Design review of the part built by this model. Coordinates are the model's own, in mm. A direction names the side the tool comes from. Round coordinates to 2 decimals unless told otherwise and drop trailing zeros. Order: outer loops, then holes, each group sorted by start corner. A loop starts at its lowest first (then second) coordinate and runs counter-clockwise, first axis right, second up. Notation, with made-up numbers: (57, 7) - (83, 7) arc R15 cw to (83, 28) - close; hole circle Ø3 at (60.25, 73). An arc over 180 degrees is marked (long way). Write item = value, one per line.
from build123d import *

# Parameters (mm, degrees)
F0_R     = 12.7
F0_R_2   = 11.176
F1_DEPTH = 7


with BuildPart() as f1:
    # F0 (on Top) → F1 (new body)
    with BuildSketch(Plane.XY):
        with BuildLine():
            Line((-34.0347428799, 10.0407234107), (-39.4287826318, 25.8310334972))
            ThreePointArc((-39.4287826318, 25.8310334972), (-49.9900963881, -1.1227458082), (-41.9203568823, -28.9243081997))
            Line((-41.9203568823, -28.9243081997), (-34.420360506, -14.0186176143))
            Line((-34.420360506, -14.0186176143), (-29.2602696984, -22.6658631364))
            Line((-29.2602696984, -22.6658631364), (-26.4620529027, -14.6181120741))
            ThreePointArc((-26.4620529027, -14.6181120741), (-14.1637665374, -14.9822916534), (-4.52611316, -22.6305667311))
            ThreePointArc((-4.52611316, -22.6305667311), (-1.6908403761, -25.8780046014), (-0.1272074495, -29.8954262311))
            ThreePointArc((-0.1272074495, -29.8954262311), (1.2367097468, -25.698504913), (3.97388684, -22.2369618714))
            ThreePointArc((3.97388684, -22.2369618714), (12.644433264, -15.5734140078), (23.5379470973, -14.6181120741))
            Line((23.5379470973, -14.6181120741), (25.7397303016, -22.8490576527))
            Line((25.7397303016, -22.8490576527), (30.579639494, -14.0186176143))
            Line((30.579639494, -14.0186176143), (38.0796431177, -28.924304553))
            ThreePointArc((38.0796431177, -28.924304553), (48.640956874, -1.9705252477), (40.5712173682, 25.8310371438))
            Line((40.5712173682, 25.8310371438), (32.0682425965, 13.0346596218))
            Line((32.0682425965, 13.0346596218), (26.9081517889, 21.6819051439))
            Line((26.9081517889, 21.6819051439), (24.1099349931, 13.6341540816))
            ThreePointArc((24.1099349931, 13.6341540816), (15.2359931939, 11.0077124587), (6.626828122, 14.4029025006))
            Line((6.626828122, 14.4029025006), (6.626828122, 27.6512976753))
            Line((6.626828122, 27.6512976753), (2.6754510519, 19.5639701469))
            ThreePointArc((2.6754510519, 19.5639701469), (-0.873171878, 21.0415739028), (-4.421794808, 19.5639701469))
            Line((-4.421794808, 19.5639701469), (-8.373171878, 27.6512976753))
            Line((-8.373171878, 27.6512976753), (-8.373171878, 14.4029025006))
            ThreePointArc((-8.373171878, 14.4029025006), (-16.5293148782, 10.0299892821), (-25.6484009718, 11.6071092754))
            Line((-25.6484009718, 11.6071092754), (-29.673149547, 19.1169503724))
            Line((-29.673149547, 19.1169503724), (-34.0347428799, 10.0407234107))
        make_face()
        Circle(F0_R, mode=Mode.SUBTRACT)
        Circle(F0_R)
        Circle(F0_R_2, mode=Mode.SUBTRACT)
    extrude(amount=F1_DEPTH)


solid = f1.part
1) We need section B-B on y = -9. Write out the cut boundary in (x, z).
Findings:
outline = (-49.66, 0) - (-6.63, 0) - (-6.63, 7) - (-49.66, 7) - close; (6.63, 0) - (47.76, 0) - (47.76, 7) - (6.63, 7) - close
2) We need section A-A on z = 1. Write out the cut boundary in (x, y).
Findings:
outline = (-41.92, -28.92) - (-34.42, -14.02) - (-29.26, -22.67) - (-26.46, -14.62) arc R19.52 cw to (-4.53, -22.63) arc R12.5 cw to (-0.13, -29.9) arc R12.5 cw to (3.97, -22.24) arc R19.52 cw to (23.54, -14.62) - (25.74, -22.85) - (30.58, -14.02) - (38.08, -28.92) arc R44.93 ccw to (40.57, 25.83) - (32.07, 13.03) - (26.91, 21.68) - (24.11, 13.63) arc R14.21 cw to (6.63, 14.4) - (6.63, 27.65) - (2.68, 19.56) arc R5 ccw to (-4.42, 19.56) - (-8.37, 27.65) - (-8.37, 14.4) arc R14.21 cw to (-25.65, 11.61) - (-29.67, 19.12) - (-34.03, 10.04) - (-39.43, 25.83) arc R44.93 ccw to start; hole circle Ø22.35 at (0, 0)
3) Clearance check with flat-ended pins moving along their axes: pin 1 Ø1 at (y, z) = (-20.5, 2) entering from +X; pin 2 Ø1.5 at (y, z) = (-18, 5.5) entering from +X; pin 3 Ø3 at (x, z) = (21.5, 3.5) entering from -Y. State where each tip first meets the part, or that it passes through.
Findings:
pin_1 = 43.96
pin_2 = 45.21
pin_3 = -14.52
4) To check wall thickness, follow L1, parallel to X at y = 12.5, z = 3.5; L2, parallel to X at y = -27, z = 6.5; L3, parallel to X at y = 1, z = 1.75. State the ranges of each line that lie inside material, in increasing order. Write a range as from..to.
Findings:
L1 = -47.22..-34.87, -32.85..-26.13, -10.53..9.49, 22.23..46.93
L2 = -43.19..-40.95, -1.09..0.63, 37.11..39.62
L3 = -49.84..-11.13, 11.13..48.68
5) We need section D-D on x = 37. Write out the cut boundary in (y, z), and give its area (3 significant figures).
Findings:
outline = (-26.78, 0) - (20.46, 0) - (20.46, 7) - (-26.78, 7) - close
area = 331 mm^2
6) The part is to be moulded in two halves that separate along X. For faces 4 (the flat face through (-36.694, 17.825, 3.451)), 5 (the flat face through (10, -7, 0)), say which applies: released by +X, released by -X, zero draft, split by the parting line, or undercut.
Findings:
face_4 = undercut
face_5 = zero draft
7) We need section C-C on x = 5. Write out the cut boundary in (y, z).
Findings:
outline = (-20.95, 0) - (-10, 0) - (-10, 7) - (-20.95, 7) - close; (10, 0) - (24.32, 0) - (24.32, 7) - (10, 7) - close
8) For faces 1 (the flat face through (-31.876, -18.282, 3.451)), 2 (the flat face through (4.679, 23.664, 3.451)), 3 (the cylindrical face through (-8.87, -6.8, 3.45)), list the 3-axis set-ups (+Z, -Z, +X, -X, +Y, -Y) from which the entire face can be reached by the end or side of a thin tool; tool diameter is ignored.
Findings:
face_1 = +Z, -Z, -Y
face_2 = +Z, -Z, +Y
face_3 = +Z, -Z
